Geometry check sheet. Reference: drawing and pictorial views, mm from the part's lowest x, y, z. A direction names the side the tool comes from. Round coordinates to 2 decimals unless told otherwise and drop trailing zeros. Loops run counter-clockwise (first coordinate to the right, second up) from the corner with the lowest first, then second, coordinate; pieces in that order, holes last. Notation, with made-up numbers: (85.5, 78.5) - (143.5, 78.5) arc R17 ccw to (143.5, 89.5) - close; hole circle Ø10 at (71.25, 3). An arc over 180 degrees is marked (long way). Answer in a Markdown table with one row per item. Add a question column.
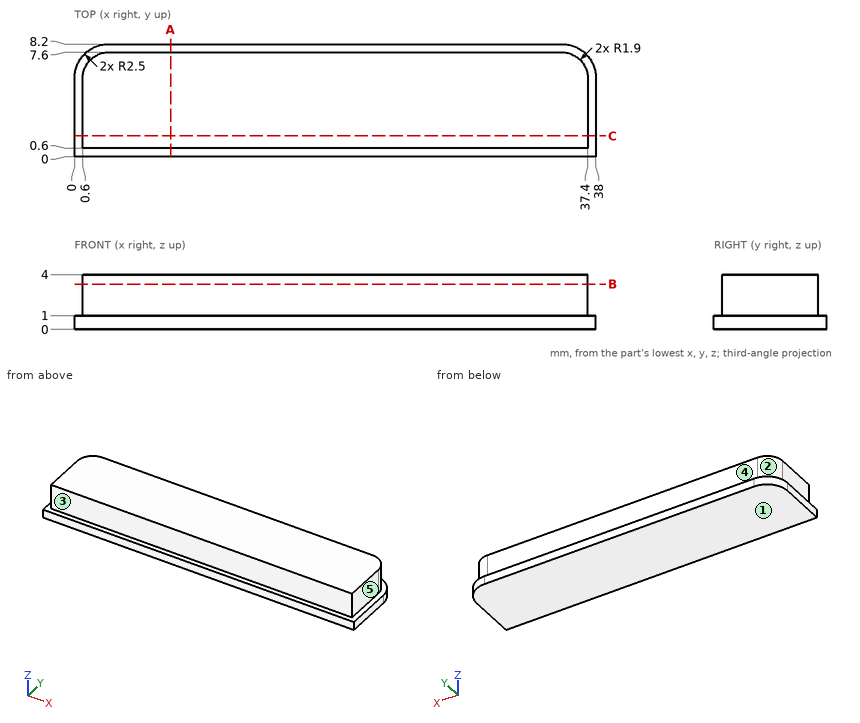
Q1. Depth check by flat-ended pin: P1, Ø1.5, axis at x = 14, z = 3, coming from the +Y side; P2, Ø1, axis at y = 7, z = 2, coming from the +X side. Enter the tip coordinate at first touch or a pass-through.
Q2. Cross-section at B-B, the plane z = 3.3. Enter the section's corners in (x, y), plus the area to 3 significant figures.
Q3. Set-up check for the marked faces 1, 2, 3, 4 and 5: record each of +Z, -Z, +X, -X, +Y, -Y from which the full face is reachable in a straight line by a thin tool's end or side.
Q4. Scan lines: line 1 (Y direction, x = 10.5, z = 3.65); line 2 (X direction, y = 3.25, z = 1.65); line 3 (Y direction, x = 2, z = 3.8). Record each from-to range of solid material in increasing order. Write a range as from..to.
Q5. Cross-section at C-C, the plane y = 1.5. Enter the section's corners in (x, z), plus the area to 3 significant figures.
Q6. Cross-section at A-A, the plane x = 7. Enter the section's corners in (y, z).
Check sheet entries:
| question | item | result |
|---|---|---|
| 1 | P1 | y = 7.6 |
| 1 | P2 | x = 37.22 |
| 2 | outline | (0.6, 0.6) - (37.4, 0.6) - (37.4, 5.7) arc R1.9 ccw to (35.5, 7.6) - (2.5, 7.6) arc R1.9 ccw to (0.6, 5.7) - close |
| 2 | area | 256 mm² |
| 3 | face 1 | -Z, +X, -X, +Y, -Y |
| 3 | face 2 | +Z, -X, +Y |
| 3 | face 3 | +Z, +X, -X, -Y |
| 3 | face 4 | +Z, +X, -X, +Y |
| 3 | face 5 | +Z, +X, +Y, -Y |
| 4 | line 1 | 0.6..7.6 |
| 4 | line 2 | 0.6..37.4 |
| 4 | line 3 | 0.6..7.53 |
| 5 | outline | (0, 0) - (38, 0) - (38, 1) - (37.4, 1) - (37.4, 4) - (0.6, 4) - (0.6, 1) - (0, 1) - close |
| 5 | area | 148 mm² |
| 6 | outline | (0, 0) - (8.2, 0) - (8.2, 1) - (7.6, 1) - (7.6, 4) - (0.6, 4) - (0.6, 1) - (0, 1) - close |
